The listing builds one solid part. Answer for the finished solid, in the listing's coordinates (mm). Face numbers are marked on the shaded views. A direction names the side the tool comes from. Round coordinates to 2 decimals unless told otherwise and drop trailing zeros. Write each loop counter-clockwise with the first axis right and the second up, starting at its lowest first coordinate (ties: lowest second). Pieces come first, ordered by that corner, then holes. Notation, with made-up numbers: M 28,72.25 L 60,72.25 A11 cw 60,81.25 Z; hole C 14,-23.5 d1. An arc over 180 degrees is marked long. One line per item, written item: value. Start each with the question number.
(1) For the marked faces 1 and 2, determine the directions among +Z, -Z, +X, -X, +Y, -Y from which every point of the face is accessible in a straight line to the end or side of a thin tool.
(2) Given P1, Ø3, axis at x = -18.5, z = 6, coming from the -Y side; P2, Ø1.2, axis at x = -32, y = 2, coming from the +Z side; P3, Ø2, axis at y = 2.5, z = 9, coming from the -X side; P4, Ø1.5, axis at y = 0.5, z = 7.5, coming from the -X side, each flat-ended and moving along its own axis, determine where each tip first touches the part or whether it passes through.
(3) Section C-C (y = 0.45) is taken. Determine the outline of the cut face in (x, z).
(4) Section D-D (z = 9) is taken. Determine the outline of the cut face in (x, y).
(5) Consider probe 1 along Y at (x, z) = (-32, 4.2); probe 2 along X at (y, z) = (2, 3.7); probe 3 along X at (y, z) = (0.6, 2.25). Determine where each line is inside the solid, lowest interval first.
(6) Section B-B (y = 2.6) is taken. Determine the outline of the cut face in (x, z).
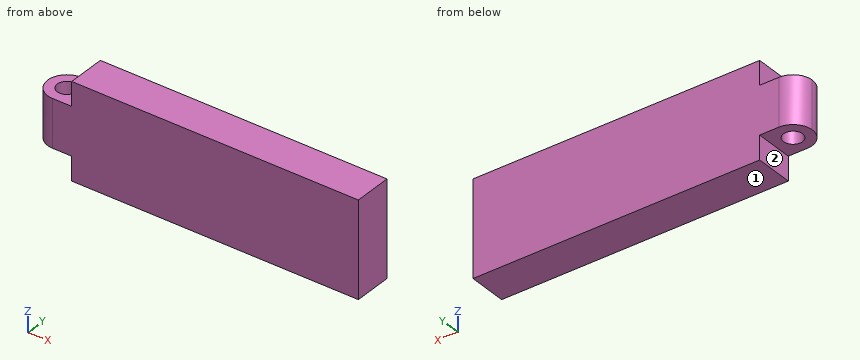
Autodesk Inventor part; units mm, degrees
ref_plane "YZ Plane" through (0, 0, 0) normal (1, 0, 0) x (0, 1, 0)
ref_plane "XZ Plane" through (0, 0, 0) normal (0, 1, 0) x (-1, 0, 0)
ref_plane "XY Plane" through (0, 0, 0) normal (0, 0, 1) x (1, 0, 0)
sketch "スケッチ1" plane through (0, 0, 0) normal (0, 1, 0) x (-1, 0, 0)
  line L0 (0, 0) -> (30, 0)
  line L1 (30, 10) -> (0, 10)
  line L2 (0, 10) -> (0, 0)
  line L3 (30, 7.5) -> (34, 7.5)
  line L4 (34, 7.5) -> (34, 2.5)
  line L5 (34, 2.5) -> (30, 2.5)
  line L6 (30, 10) -> (30, 7.5)
  line L7 (30, 2.5) -> (30, 0)
  dimension "d0" = 30
  dimension "d1" = 10
  dimension "d5" = 5
  dimension "d6" = 2.5
extrude "押し出し1" add sketch "スケッチ1" along normal blind 4
sketch "スケッチ2" plane through (0, 0, 0) normal (0, 0, 1) x (1, 0, 0)
  circle A0 centre (-32, 2) radius 1
  line L0 (-34, 4) -> (-30, 4)
  line L1 (-34, 0) -> (-34, 4)
  point P0 (0, 0)
  dimension "d7" = 2
  dimension "d8" = 2
  dimension "d9" = 2
extrude "押し出し2" cut sketch "スケッチ2" along normal blind 10
fillet "フィレット1" radius 2 1 edges at (-34, 0, 5)
fillet "フィレット2" radius 2 1 edges at (-34, 4, 5)
properties part number "promo3"
Recorded:
1. face 1: -Z, +X, -X, +Y, -Y
1. face 2: -Z, -X, +Y, -Y
2. P1: stops at y = 0
2. P2: passes through
2. P3: stops at x = -30
2. P4: stops at x = -33.85
3. outline: M -33.26,2.5 L -30,2.5 L -30,0 L 0,0 L 0,10 L -30,10 L -30,7.5 L -33.26,7.5 Z
4. outline: M -30,0 L 0,0 L 0,4 L -30,4 Z
5. probe 1: y = 0 to 1, 3 to 4
5. probe 2: x = -34 to -33, -31 to 0
5. probe 3: x = -30 to 0
6. outline: M -33.91,2.5 L -32.8,2.5 L -32.8,7.5 L -33.91,7.5 Z; M -31.2,2.5 L -30,2.5 L -30,0 L 0,0 L 0,10 L -30,10 L -30,7.5 L -31.2,7.5 Z
